```python
from build123d import *

# Parameters (mm, degrees)
BOSS_EXTRUDE1_DEPTH = 15
SKETCH2_R           = 2.5
BOSS_EXTRUDE2_DEPTH = 1.2
SKETCH3_W           = 0.2
SKETCH3_H           = 1.5
BOSS_EXTRUDE3_DEPTH = 2
SKETCH4_W           = 1.4
SKETCH4_H           = 2
CUT_EXTRUDE1_DEPTH  = 1.5
BOSS_EXTRUDE4_DEPTH = 9
BOSS_EXTRUDE5_DEPTH = 10.5
SKETCH7_R           = 2
BOSS_EXTRUDE6_DEPTH = 0.5
SKETCH8_R           = 0.5
CUT_EXTRUDE2_DEPTH  = 4.5


with BuildPart() as part:
    # Sketch1 → Boss-Extrude1 (new body)
    with BuildSketch(Plane(origin=(0, 0, 0), x_dir=(1, 0, 0), z_dir=(0, 1, 0))):
        with BuildLine():
            Line((-3.31662479, 5), (3.31662479, 5))
            ThreePointArc((3.31662479, 5), (6, 0), (3.31662479, -5))
            Line((3.31662479, -5), (-3.31662479, -5))
            ThreePointArc((-3.31662479, -5), (-6, 0), (-3.31662479, 5))
        make_face()
    extrude(amount=BOSS_EXTRUDE1_DEPTH)

    # Sketch2 → Boss-Extrude2 (add)
    with BuildSketch(Plane.XZ):
        with Locations(Location((0, 0, 0), (0, 0, 270))):
            Circle(SKETCH2_R)
    extrude(amount=BOSS_EXTRUDE2_DEPTH)

    # Sketch3 → Boss-Extrude3 (add)
    with BuildSketch(Plane.XZ):
        with Locations((4, 0)):
            Rectangle(SKETCH3_W, SKETCH3_H)
        with Locations((-4, 0)):
            Rectangle(SKETCH3_W, SKETCH3_H)
    extrude(amount=BOSS_EXTRUDE3_DEPTH)

    # Sketch4 → Cut-Extrude1 (cut)
    with BuildSketch(Plane.XZ):
        with Locations((-5.3, 0)):
            Rectangle(SKETCH4_W, SKETCH4_H)
        with Locations((5.3, 0)):
            Rectangle(SKETCH4_W, SKETCH4_H)
    extrude(amount=-CUT_EXTRUDE1_DEPTH, mode=Mode.SUBTRACT)

    # Sketch5 → Boss-Extrude4 (add)
    with BuildSketch(Plane(origin=(0, 15, 0), x_dir=(1, 0, 0), z_dir=(0, 1, 0))):
        with BuildLine():
            Line((-5, 5), (5, 5))
            ThreePointArc((5, 5), (5.707106781, 4.707106781), (6, 4))
            Line((6, 4), (6, -4))
            ThreePointArc((6, -4), (5.707106781, -4.707106781), (5, -5))
            Line((5, -5), (-5, -5))
            ThreePointArc((-5, -5), (-5.707106781, -4.707106781), (-6, -4))
            Line((-6, -4), (-6, 4))
            ThreePointArc((-6, 4), (-5.707106781, 4.707106781), (-5, 5))
        make_face()
    extrude(amount=BOSS_EXTRUDE4_DEPTH)

    # Sketch6 → Boss-Extrude5 (add)
    with BuildSketch(Plane(origin=(0, 24, 0), x_dir=(1, 0, 0), z_dir=(0, 1, 0))):
        with BuildLine():
            Line((-1.118033989, 1), (1.118033989, 1))
            ThreePointArc((1.118033989, 1), (0, -1.5), (-1.118033989, 1))
        make_face()
    extrude(amount=BOSS_EXTRUDE5_DEPTH)

    # Sketch7 → Boss-Extrude6 (add)
    with BuildSketch(Plane(origin=(0, 24, 0), x_dir=(1, 0, 0), z_dir=(0, 1, 0))):
        with Locations(Location((0, 0, 0), (0, 0, 90))):
            Circle(SKETCH7_R)
    extrude(amount=BOSS_EXTRUDE6_DEPTH)

    # Sketch8 → Cut-Extrude2 (cut)
    with BuildSketch(Plane(origin=(0, 24, 0), x_dir=(1, 0, 0), z_dir=(0, 1, 0))):
        with Locations(Location((-4.5, 0, 0), (0, 0, 270))):
            Circle(SKETCH8_R)
        with Locations(Location((4.5, 0, 0), (0, 0, 90))):
            Circle(SKETCH8_R)
    extrude(amount=-CUT_EXTRUDE2_DEPTH, mode=Mode.SUBTRACT)


solid = part.part
```
Geometry: final body of the model. Coordinates: model frame, mm. A direction names the side the tool comes from. Round coordinates to 2 decimals unless told otherwise and drop trailing zeros. Order: outer loops, then holes, each group sorted by start corner. A loop starts at its lowest first (then second) coordinate and runs counter-clockwise, first axis right, second up. Notation, with made-up numbers: (49, 40.25) - (64, 40.25) arc R18 ccw to (64, 54.25) - close; hole circle Ø7 at (29, 9). An arc over 180 degrees is marked (long way). Write item = value, one per line. Start each with the question number.
Q1. Cut plane C-C on y = 0.5. Return the cut outline in (x, z), and give its area (3 significant figures).
Q2. Access query for faces 1 (the flat face through (-3.9, -1, 0)), 2 (the flat face through (-5, 15, -4)), 3 (the flat face through (5, 1, 1)), 4 (the flat face through (0, 24.5, -1.3)). Directions: +Z, -Z, +X, -X, +Y, -Y. A direction counts if a zero-diameter tool reaches every point of the face in a straight line with its end or side. Return the directions, or none.
Q3. Cut plane B-B on x = 0. Return the cut outline in (y, z).
Q4. Pull-direction query (Z, two-part tool) for faces 5 (the flat face through (4.6, 1, 0)), 6 (the cylindrical face through (-6, 7, 0)), 7 (the flat face through (0, 12, -5)), 8 (the flat face through (-5, 15, 4)); classes: +Z half, -Z half, draft (parallel to the pull), parting line (faces both ways), or undercut.
Q5. Pin query (flat end, axial travel): pin 1 (1.3 mm diameter, centred on x = -4, z = -2.5, fed in from -Y); pin 2 (1.2 mm diameter, centred on y = -1, z = 0, fed in from -X); pin 3 (1.1 mm diameter, centred on x = -5.5, z = 0, fed in from -Y); pin 4 (2 mm diameter, centred on x = -4.5, z = 1.5, fed in from -Y). Return the tip coordinate at first contact, or that it passes through.
Q6. Ray query, line 1 (X direction, y = 22.7, z = 0); line 2 (Z direction, x = 4.5, y = 20.95); line 3 (Y direction, x = 3.75, z = -0.25). Return the intervals inside material, ascending. Write a range as from..to.
Q7. Cut plane A-A on y = 20.5. Return the cut outline in (x, z), and give its area (3 significant figures).
Outcome:
q1.outline = (-5.92, -1) arc R6 ccw to (-3.32, -5) - (3.32, -5) arc R6 ccw to (5.92, -1) - (4.6, -1) - (4.6, 1) - (5.92, 1) arc R6 ccw to (3.32, 5) - (-3.32, 5) arc R6 ccw to (-5.92, 1) - (-4.6, 1) - (-4.6, -1) - close
q1.area = 98.6 mm^2
q2.face_1 = +Z, -Z, -Y
q2.face_2 = -Z, -X, -Y
q2.face_3 = +X, -Y
q2.face_4 = +Y
q3.outline = (-1.2, -2.5) - (0, -2.5) - (0, -5) - (24, -5) - (24, -2) - (24.5, -2) - (24.5, -1) - (34.5, -1) - (34.5, 1.5) - (24.5, 1.5) - (24.5, 2) - (24, 2) - (24, 5) - (0, 5) - (0, 2.5) - (-1.2, 2.5) - close
q4.face_5 = undercut
q4.face_6 = parting line
q4.face_7 = -Z half
q4.face_8 = draft
q5.pin_1 = 0
q5.pin_2 = -4.1
q5.pin_3 = 1.5
q5.pin_4 = -2
q6.line_1 = -6..-5, -4..4, 5..6
q6.line_2 = -5..-0.5, 0.5..5
q6.line_3 = 0..24
q7.outline = (-6, -4) arc R1 ccw to (-5, -5) - (5, -5) arc R1 ccw to (6, -4) - (6, 4) arc R1 ccw to (5, 5) - (-5, 5) arc R1 ccw to (-6, 4) - close; hole circle Ø1 at (-4.5, 0); hole circle Ø1 at (4.5, 0)
q7.area = 118 mm^2
